from build123d import *

# Parameters (mm, degrees)
BOSS_EXTRUDE1_DEPTH  = 4
SKETCH2_W            = 8
SKETCH2_H            = 8
BOSS_EXTRUDE2_DEPTH  = 26
BOSS_EXTRUDE3_DEPTH  = 7
BOSS_EXTRUDE4_DEPTH  = 6
M3_CLEARANCE_HOLE1_D = 3.2
M3_CLEARANCE_HOLE2_D = 3.2


with BuildPart() as part:
    # Sketch1 → Boss-Extrude1 (new body)
    with BuildSketch(Plane(origin=(0, 0, 0), x_dir=(0, 0, -1), z_dir=(1, 0, 0))):
        Polygon((0, 0), (-8, 0), (-8, -8), (178, -8), (178, 0), (170, 0), align=None)
    extrude(amount=BOSS_EXTRUDE1_DEPTH)

    # Sketch2 → Boss-Extrude2 (add)
    with BuildSketch(Plane(origin=(4, 0, 0), x_dir=(0, 0, -1), z_dir=(1, 0, 0))):
        with Locations((-4, -4)):
            Rectangle(SKETCH2_W, SKETCH2_H)
        with Locations((174, -4)):
            Rectangle(SKETCH2_W, SKETCH2_H)
    extrude(amount=BOSS_EXTRUDE2_DEPTH)

    # Sketch1<2> → Boss-Extrude3 (add)
    with BuildSketch(Plane(origin=(0, 0, 0), x_dir=(0, 0, -1), z_dir=(1, 0, 0))):
        Polygon((0, 0), (-8, 0), (-8, -8), (178, -8), (178, 0), (170, 0), align=None)
    extrude(amount=-BOSS_EXTRUDE3_DEPTH)

    # Sketch4 → Boss-Extrude4 (add)
    with BuildSketch(Plane.ZY.offset(7)):
        Polygon((-178, 0), (-178, 60), (-162, 60), (-162, 0), (8, 0), (8, -8), (-178, -8), align=None)
    extrude(amount=BOSS_EXTRUDE4_DEPTH)

    # M3 Clearance Hole1 (through all)
    with Locations(Plane.ZX):
        with Locations((0, 0)):
            Hole(M3_CLEARANCE_HOLE1_D / 2)

    # M3 Clearance Hole2 (through all)
    with Locations(Plane(origin=(-7, 52, -170), x_dir=(0, 0, 1), z_dir=(1, 0, 0))):
        with Locations((0, 0)):
            Hole(M3_CLEARANCE_HOLE2_D / 2)


solid = part.part
Read the model definition and answer for the solid it produces. Units are mm, in the model's axes. A direction names the side the tool comes from. Coordinates: 2 decimals unless noted, no trailing zeros. Order: outer loops, then holes, each group sorted by start corner. A loop starts at its lowest first (then second) coordinate and runs counter-clockwise, first axis right, second up. Notation, with made-up numbers: (50, -18) -> (101, -18) arc R19 ccw to (101, -1) -> close; hole circle Ø2 at (82, 24). An arc over 180 degrees is marked (long way). Answer as a JSON object with one key per item and string values.
1) A tool of negligible diameter and unlimited length cuts with its end or side. For faces 4 (the face through (-10, 30, -162)), 5 (the face through (-7, 30, -170)), 6 (the face through (17, -4, -170)), from which of +Z, -Z, +X, -X, +Y, -Y can it reach the whole face along a straight path? Write none if from no direction.
Model answer:
{"face 4": "+Z, +X, -X, +Y", "face 5": "+Z, -Z, +X, +Y", "face 6": "+X, +Y, -Y"}
2) The mould has two halves that part along X. Classify faces 1 (the face through (-13, -2, -119)), 2 (the face through (-10.04, 52.61, -171.48)), 3 (the face through (-0.97, -4.06, 1.27)): released by +X, released by -X, zero draft, split by the parting line, or undercut.
Model answer:
{"face 1": "released by -X", "face 2": "zero draft", "face 3": "undercut"}
3) Consider line 1 along Y through (x, z) = (-11.15, -170); line 2 along Z through (x, y) = (-9, 52); line 3 along Y through (x, z) = (-5.5, -55). Determine where each line is inside the solid, lowest interval first. Write a range as from..to.
Model answer:
{"line 1": "y = -8..50.4, 53.6..60", "line 2": "z = -178..-171.6, -168.4..-162", "line 3": "y = -8..0"}
4) A cutting plane is placed at A-A, the plane x = 10.5. Determine the outline of the cut face in (y, z), plus the area to 3 significant figures.
Model answer:
{"outline": "(-8, -178) -> (0, -178) -> (0, -170) -> (-8, -170) -> close; (-8, 0) -> (0, 0) -> (0, 8) -> (-8, 8) -> close", "area": "128 mm²"}
5) A cutting plane is placed at C-C, the plane z = -23.5. Determine the outline of the cut face in (x, y), plus the area to 3 significant figures.
Model answer:
{"outline": "(-13, -8) -> (4, -8) -> (4, 0) -> (-13, 0) -> close", "area": "136 mm²"}
6) Each of these flat-tipped pins is pushed along its axis until it touches: pin 1 (4 mm diameter, centred on y = 52, z = -170, fed in from -X); pin 2 (6.5 mm diameter, centred on y = -2, z = -52.5, fed in from +X); pin 3 (3 mm diameter, centred on x = -1.5, z = -120.5, fed in from +Y); pin 4 (6.5 mm diameter, centred on x = -11, y = 18, fed in from +Z). Where does it stop, or does it pass through?
Model answer:
{"pin 1": "stops at x = -13", "pin 2": "stops at x = 4", "pin 3": "stops at y = 0", "pin 4": "stops at z = -162"}
7) A cutting plane is placed at B-B, the plane y = 39.5. Determine the outline of the cut face in (x, z), plus the area to 3 significant figures.
Model answer:
{"outline": "(-13, -178) -> (-7, -178) -> (-7, -162) -> (-13, -162) -> close", "area": "96.0 mm²"}
